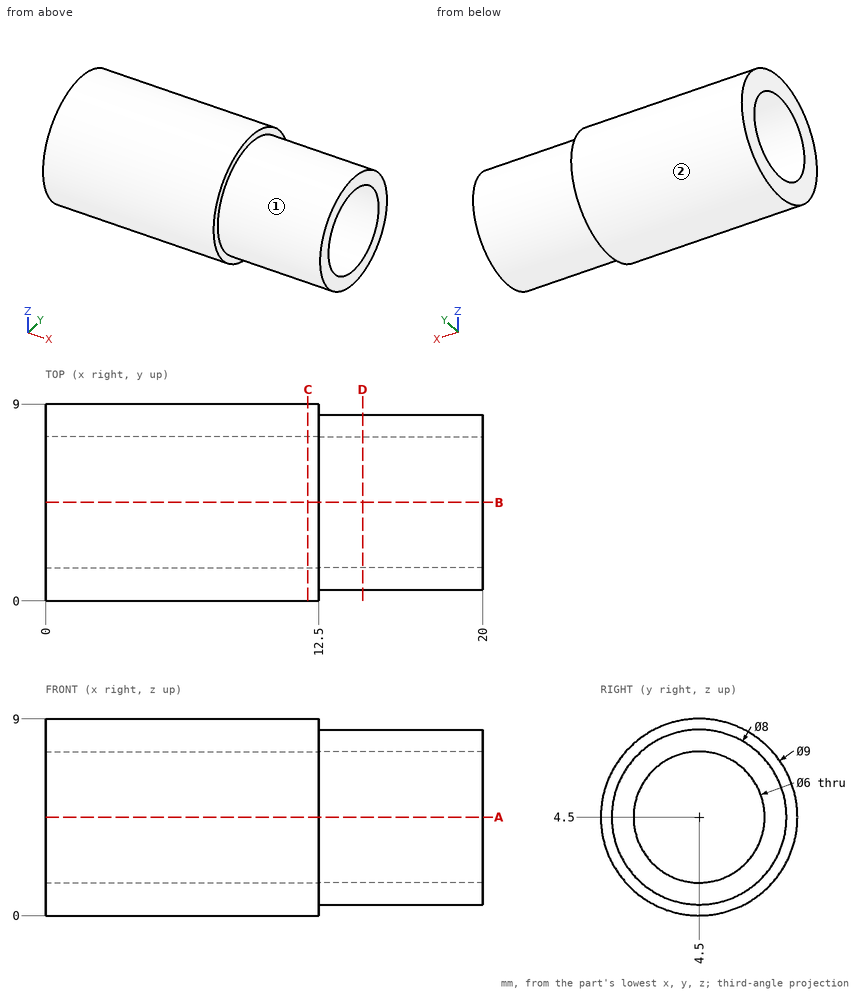
Study the drawing (mm; zero at the part's minimum x, y, z) and answer. A direction names the side the tool comes from. Round coordinates to 2 decimals unless told otherwise and drop trailing zeros. Write each loop counter-clockwise with the first axis right and the second up, starting at its lowest first coordinate (ties: lowest second). Pieces come first, ordered by that corner, then holes. Notation, with made-up numbers: (59, 39.5) - (94, 39.5) arc R8 ccw to (94, 49.5) - close; hole circle Ø11 at (-27, 32.25). An arc over 180 degrees is marked (long way). Use a Markdown table: item, result. Add a question column.
1. Consider line 1 (Z direction, x = 18, y = 4.5); line 2 (Z direction, x = 2.75, y = 4.5); line 3 (X direction, y = 8.5, z = 5.25). Determine where each line is inside the solid, lowest interval first.
2. The part is cut by section C-C (x = 12). Write down the section's boundary in (y, z), and give its area (3 significant figures).
3. Flat-ended cylindrical pins translate along their axes: P1, Ø1, axis at x = 7, y = 1, coming from the -Z side; P2, Ø5, axis at y = 4.5, z = 4.5, coming from the +X side. Find the tip coordinate at first contact, or state that the pin passes through.
4. The part is cut by section D-D (x = 14.5). Write down the section's boundary in (y, z).
5. A tool of negligible diameter and unlimited length cuts with its end or side. For the marked faces 1 and 2, from which of +Z, -Z, +X, -X, +Y, -Y can it reach the whole face along a straight path? Write none if from no direction.
6. The part is cut by section A-A (z = 4.5). Write down the section's boundary in (x, y), and give its area (3 significant figures).
Reported:
| question | item | result |
|---|---|---|
| 1 | line 1 | 0.5 to 1.5, 7.5 to 8.5 |
| 1 | line 2 | 0 to 1.5, 7.5 to 9 |
| 1 | line 3 | 0 to 12.5 |
| 2 | outline | circle Ø9 at (4.5, 4.5); hole circle Ø6 at (4.5, 4.5) |
| 2 | area | 35.3 mm^2 |
| 3 | P1 | z = 1.15 |
| 3 | P2 | through |
| 4 | outline | circle Ø8 at (4.5, 4.5); hole circle Ø6 at (4.5, 4.5) |
| 5 | face 1 | +X |
| 5 | face 2 | +X, -X |
| 6 | outline | (0, 0) - (12.5, 0) - (12.5, 0.5) - (20, 0.5) - (20, 1.5) - (0, 1.5) - close; (0, 7.5) - (20, 7.5) - (20, 8.5) - (12.5, 8.5) - (12.5, 9) - (0, 9) - close |
| 6 | area | 52.5 mm^2 |
